Verification items for the finished model (mm, model axes). A direction names the side the tool comes from. Give positions to 0.01 mm unless a question says otherwise; leave off trailing zeros. Loops run counter-clockwise (first coordinate to the right, second up) from the corner with the lowest first, then second, coordinate; pieces in that order, holes last. Notation, with made-up numbers: (40, -1.5) - (99, -1.5) arc R7 ccw to (99, 4.5) - close; hole circle Ø3 at (48.25, 71.25). An arc over 180 degrees is marked (long way). One line per question, with ' | ' between items. Start each with the question number.
1. Thickness scan on line 1 along X through (y, z) = (1.7, 0); line 2 along Y through (x, z) = (-62, 6.5); line 3 along Z through (x, y) = (1, 1.85). Record the ranges inside material, lowest first. Write a range as from..to.
2. Tool access check on faces 1 (the face through (-60, 1.8, 14)), 2 (the face through (-70.079, 0.406, 70.278)). Record the directions out of +Z, -Z, +X, -X, +Y, -Y that give a thin tool (end or side, any length) a straight path to the whole face; none if there is none.
3. Mould release check, pull along X, two halves, no side actions. Record for faces 3 (the face through (2.64, 1.17, -59.94)), 4 (the face through (-35, 0.8, -52)), 5 (the face through (-37.99, 2.053, -49.546)): +X half, -X half, draft (parallel to the pull), parting line (faces both ways), or undercut.
4. Section check A-A, the plane x = 0. Enter the section's corners in (y, z).
5. Depth check by flat-ended pin: pin 1 Ø6 at (x, z) = (60, -44) entering from +Y; pin 2 Ø5 at (x, z) = (67.88, -67.88) entering from -Y; pin 3 Ø1 at (y, z) = (1.5, 14.5) entering from -X. Enter the tip coordinate at first touch or a pass-through.
6. Section check B-B, the plane z = 0. Enter the section's corners in (x, y), then the cut area to 3 significant figures.
7. Section check C-C, the plane y = 1.4. Enter the section's corners in (x, z), then the cut area to 3 significant figures.
from build123d import *

# Parameters (mm, degrees)
CROQUIS1_W              = 154.2
CROQUIS1_H              = 154.2
SALIENTE_EXTRUIR1_DEPTH = 0.8
CROQUIS2_R              = 60
CORTAR_EXTRUIR1_DEPTH   = 110.038800434
SALIENTE_EXTRUIR2_START = 1
CROQUIS3_R              = 60.995810587
CROQUIS3_R_2            = 60
SALIENTE_EXTRUIR2_DEPTH = 1
SALIENTE_EXTRUIR3_START = 0.5
CROQUIS4_R              = 62.434019261
CROQUIS4_R_2            = 60
SALIENTE_EXTRUIR3_DEPTH = 0.5
CROQUIS5_R              = 3.25
CORTAR_EXTRUIR2_DEPTH   = 110.046182877


with BuildPart() as part:
    # Croquis1 → Saliente-Extruir1 (new body)
    with BuildSketch(Plane(origin=(0, 0, 0), x_dir=(1, 0, 0), z_dir=(0, 1, 0))):
        Rectangle(CROQUIS1_W, CROQUIS1_H)
    extrude(amount=SALIENTE_EXTRUIR1_DEPTH)

    # Croquis2 → Cortar-Extruir1 (cut, through all)
    with BuildSketch(Plane(origin=(0, 0.8, 0), x_dir=(1, 0, 0), z_dir=(0, 1, 0))):
        with Locations(Location((0, 0, 0), (0, 0, 270))):
            Circle(CROQUIS2_R)
    extrude(amount=-CORTAR_EXTRUIR1_DEPTH, mode=Mode.SUBTRACT)

    # Croquis3 → Saliente-Extruir2 (add)
    with BuildSketch(Plane(origin=(0, 0.8, 0), x_dir=(1, 0, 0), z_dir=(0, 1, 0)).offset(SALIENTE_EXTRUIR2_START)):
        with Locations(Location((0, 0, 0), (0, 0, 90))):
            Circle(CROQUIS3_R)
        with Locations(Location((0, 0, 0), (0, 0, 270))):
            Circle(CROQUIS3_R_2, mode=Mode.SUBTRACT)
    extrude(amount=-SALIENTE_EXTRUIR2_DEPTH)

    # Croquis4 → Saliente-Extruir3 (add)
    with BuildSketch(Plane(origin=(0, 1.8, 0), x_dir=(1, 0, 0), z_dir=(0, 1, 0)).offset(SALIENTE_EXTRUIR3_START)):
        with Locations(Location((0, 0, 0), (0, 0, 270))):
            Circle(CROQUIS4_R)
        with Locations(Location((0, 0, 0), (0, 0, 270))):
            Circle(CROQUIS4_R_2, mode=Mode.SUBTRACT)
    extrude(amount=-SALIENTE_EXTRUIR3_DEPTH)

    # Croquis5 → Cortar-Extruir2 (cut, through all)
    with BuildSketch(Plane(origin=(0, 0.8, 0), x_dir=(1, 0, 0), z_dir=(0, 1, 0))):
        with Locations(Location((-67.882250994, 67.882250994, 0), (0, 0, 270))):
            Circle(CROQUIS5_R)
        with Locations(Location((67.882250994, 67.882250994, 0), (0, 0, 90))):
            Circle(CROQUIS5_R)
        with Locations(Location((-67.882250994, -67.882250994, 0), (0, 0, 90))):
            Circle(CROQUIS5_R)
        with Locations(Location((67.882250994, -67.882250994, 0), (0, 0, 270))):
            Circle(CROQUIS5_R)
    extrude(amount=-CORTAR_EXTRUIR2_DEPTH, mode=Mode.SUBTRACT)


solid = part.part
Results list:
1) line 1: -61..-60, 60..61 | line 2: 0..0.8, 1.8..2.3 | line 3: -62.43..-59.99, 59.99..62.43
2) face 1: none | face 2: +Y, -Y
3) face 3: undercut | face 4: draft | face 5: parting line
4) outline: (0, -77.1) - (0.8, -77.1) - (0.8, -61) - (1.8, -61) - (1.8, -62.43) - (2.3, -62.43) - (2.3, -60) - (0, -60) - close; (0, 60) - (2.3, 60) - (2.3, 62.43) - (1.8, 62.43) - (1.8, 61) - (0.8, 61) - (0.8, 77.1) - (0, 77.1) - close
5) pin 1: y = 0.8 | pin 2: through | pin 3: x = -60.82
6) outline: (-77.1, 0) - (-60, 0) - (-60, 2.3) - (-62.43, 2.3) - (-62.43, 1.8) - (-61, 1.8) - (-61, 0.8) - (-77.1, 0.8) - close; (60, 0) - (77.1, 0) - (77.1, 0.8) - (61, 0.8) - (61, 1.8) - (62.43, 1.8) - (62.43, 2.3) - (60, 2.3) - close | area: 31.8 mm²
7) outline: circle Ø121.99 at (0, 0); hole circle Ø120 at (0, 0) | area: 379 mm²
